Here's how the part is built. I have some questions about the finished solid (model axes, mm). A direction names the side the tool comes from. Coordinates: 2 decimals unless noted, no trailing zeros. Loops run counter-clockwise (first coordinate to the right, second up) from the corner with the lowest first, then second, coordinate; pieces in that order, holes last. Notation, with made-up numbers: M 71,39 L 81,39 A7 cw 81,49 Z; hole C 11,-28 d4. An arc over 180 degrees is marked long. Use one line per item in the form item = value. Start each with the question number.
(1) On a 3-axis mill with a long thin cutter (end or side, diameter ignored), from which of +Z, -Z, +X, -X, +Y, -Y can I reach the whole of each face in a straight line? I mean faces 4 (the flat face through (-5.937, -32, 15)), 5 (the flat face through (4, -24.621, 15)), 6 (the flat face through (-4, 2.779, 15)). Say none if no direction works.
(2) Imagine slicing it at A-A, the plane x = 0. Please give me the cut outline in (y, z), and give its area (3 significant figures).
(3) Please list where these lines run through material, in increasing order: L1, parallel to Y at x = -11, z = 4.75; L2, parallel to X at y = -27, z = 27; L3, parallel to X at y = -11, z = 25.
(4) Imagine slicing it at C-C, the plane z = 6. State how many separate pieces and enclosed holes the cut face has, and give its area (3 significant figures).
(5) Thinking about a two-plate mould opening in X: for faces 1 (the cylindrical face through (-3.39, 3.35, 29.4)), 2 (the flat face through (-5, -39.621, 15)), 3 (the cylindrical face through (15.111, -21.614, 15.21)), which applies, +X half, -X half, draft (parallel to the pull), parting line (faces both ways), or undercut?
(6) Imagine slicing it at D-D, the plane x = -10.5. Please give me the cut outline in (y, z), and give its area (3 significant figures).
(7) Imagine slicing it at B-B, the plane y = -26.5. Please give me the cut outline in (x, z).
(8) Will these pins go through, and if not, where does the flat tip stop? P1, Ø7.5, axis at y = -35, z = 8, coming from the -X side; P2, Ø3.5, axis at y = -31.87, z = 24, coming from the +X side; P3, Ø3.5, axis at x = 3, z = 17, coming from the -Y side.
```python
from build123d import *

# Parameters (mm, degrees)
F0_W     = 2.4
F0_H     = 3
F0_H_2   = 15
F1_DEPTH = 30
F2_R     = 1.5
F3_DEPTH = 25
F4_R     = 2
F5_R     = 10


with BuildPart() as f1:
    # F0 (on Top) → F1 (new body)
    with BuildSketch(Plane.XY):
        Polygon((-12.036903, -21.621074), (-12.036903, 2.778926), (4.963097, 2.778926), (4.963097, -2.221074), (12.963097, -2.221074), (12.963097, -16.621074), (4.963097, -16.621074), (4.963097, -21.621074), (0.903097, -21.621074), (0.903097, -24.621074), (17.963097, -24.621074), (17.963097, 5.778926), (-15.036903, 5.778926), (-15.036903, -24.621074), (-5.936903, -24.621074), (-5.936903, -21.621074), align=None)
        with Locations((-0.296903, -23.121074)):
            Rectangle(F0_W, F0_H)
        with Locations((-0.296903, -32.121074)):
            Rectangle(F0_W, F0_H_2)
        with Locations((-4.736903, -23.121074)):
            Rectangle(F0_W, F0_H)
        with Locations((-4.736903, -32.121074)):
            Rectangle(F0_W, F0_H_2)
    extrude(amount=F1_DEPTH)

    # F2 (on face) → F3 (cut)
    with BuildSketch(Plane(origin=(-5.936903, 0, 0), x_dir=(0, -1, 0), z_dir=(-1, 0, 0))):
        with Locations((32.121074, 6)):
            Circle(F2_R)
        with Locations((31.869072, 24)):
            Circle(F2_R)
    extrude(amount=-F3_DEPTH, mode=Mode.SUBTRACT)

    # F4
    f4_edges = [f1.edges().sort_by_distance(p)[0] for p in [
        (-12.036903, -9.421074, 30),
        (-3.536903, 2.778926, 30),
        (4.963097, 0.278926, 30),
        (4.963097, -19.121074, 30),
        (1.733097, -21.621074, 30),
        (-7.786903, -21.621074, 30),
        (12.963097, -9.421074, 30),
        (-3.536903, 2.778926, 0),
        (-12.036903, -9.421074, 0),
        (-7.786903, -21.621074, 0),
        (1.733097, -21.621074, 0),
        (4.963097, -19.121074, 0),
        (4.963097, 0.278926, 0),
    ]]
    fillet(f4_edges, radius=F4_R)

    # F5
    f5_edges = [f1.edges().sort_by_distance(p)[0] for p in [
        (17.963097, 5.778926, 15),
        (17.963097, -24.621074, 15),
    ]]
    fillet(f5_edges, radius=F5_R)


solid = f1.part
```
Answer:
q1.face_4 = +Z, -Z, -X, -Y
q1.face_5 = +Z, -Z, +X, -Y
q1.face_6 = +Z, -Z
q2.outline = M -39.62,0 L -23.62,0 A2 ccw -21.62,2 L -21.62,28 A2 ccw -23.62,30 L -39.62,30 Z; M 2.78,2 A2 ccw 4.78,0 L 5.78,0 L 5.78,30 L 4.78,30 A2 ccw 2.78,28 Z; hole C -32.12,6 d3; hole C -31.87,24 d3
q2.area = 612 mm²
q3.L1 = -24.62 to -21.62, 2.78 to 5.78
q3.L2 = -5.94 to -3.54, -1.5 to 0.9
q3.L3 = -15.04 to -12.04, 12.96 to 17.96
q4.separate_pieces = 3
q4.enclosed_holes = 0
q4.area = 482 mm²
q5.face_1 = undercut
q5.face_2 = draft
q5.face_3 = +X half
q6.outline = M -24.62,0 L -23.62,0 A2 ccw -21.62,2 L -21.62,28 A2 ccw -23.62,30 L -24.62,30 Z; M 2.78,2 A2 ccw 4.78,0 L 5.78,0 L 5.78,30 L 4.78,30 A2 ccw 2.78,28 Z
q6.area = 177 mm²
q7.outline = M -5.94,0 L -3.54,0 L -3.54,30 L -5.94,30 Z; M -1.5,0 L 0.9,0 L 0.9,30 L -1.5,30 Z
q8.P1 = -5.94
q8.P2 = 0.9
q8.P3 = -24.62
